Geometry check sheet. Reference: the model listing, model coordinates, mm. Face numbers are marked on the shaded views. A direction names the side the tool comes from. Coordinates: 2 decimals unless noted, no trailing zeros. Order: outer loops, then holes, each group sorted by start corner. A loop starts at its lowest first (then second) coordinate and runs counter-clockwise, first axis right, second up. Notation, with made-up numbers: (63, -14.5) - (72, -14.5) arc R28 ccw to (72, 22.5) - close; hole circle Ø10 at (26.25, 68.25). An arc over 180 degrees is marked (long way). Return JSON: item names as keys, results as strings. Group by question number.
Item 1: Section check C-C on z = 24.5. Enter the section's corners in (x, y), then the cut area to 3 significant figures.
Item 2: Section check A-A on y = -39.5. Enter the section's corners in (x, z).
Item 3: Tool access check on the marked faces 4, 5, 6, 7 and 8. Record the directions out of +Z, -Z, +X, -X, +Y, -Y that give a thin tool (end or side, any length) a straight path to the whole face; none if there is none.
Item 4: Draft check along Z on the marked faces 1, 2 and 3. Enter one of: pulls with the +Z half, pulls with the -Z half, needs draft (parallel to the pull), parting line crosses it, or undercut.
Item 5: Gauge pin test, flat ends, axial feed: pin 1 (4 mm diameter, centred on y = -45.5, z = 1, fed in from +X); pin 2 (6 mm diameter, centred on x = 35.5, z = 10, fed in from +Y); pin 3 (7.5 mm diameter, centred on y = -35.5, z = 40.5, fed in from +X); pin 4 (7.5 mm diameter, centred on x = 36, y = -36.5, fed in from +Z). Record the tip position at first contact, or that the pin passes through.
Item 6: Section check B-B on x = 27. Enter the section's corners in (y, z).
Item 7: Scan lines: probe 1 along X at (y, z) = (-31, 33); probe 2 along Z at (x, y) = (37, -11); probe 3 along Z at (x, y) = (7, -4). Record each from-to range of solid material in increasing order.
Item 8: Section check D-D on z = 45. Enter the section's corners in (x, y), then the cut area to 3 significant figures.
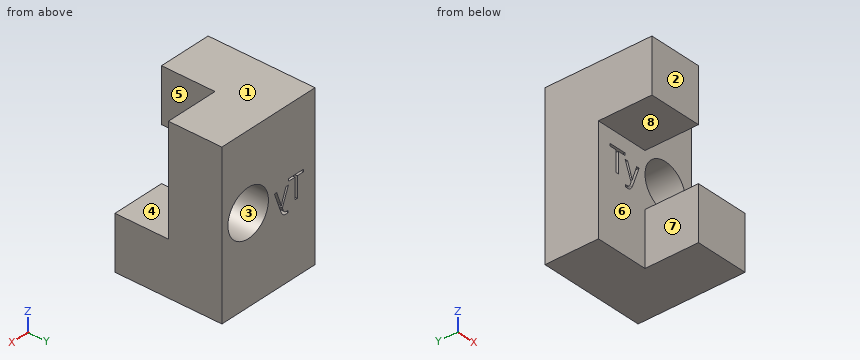
from build123d import *

# Parameters (mm, degrees)
F0_W     = 25.4
F0_H     = 25.4
F1_DEPTH = 50.8
F2_R     = 11.0649221301
F3_DEPTH = 25.4
F4_W     = 25.4
F4_H     = 25.4
F5_DEPTH = 50.8


with BuildPart() as f1:
    # F0 (on Front) → F1 (new body)
    with BuildSketch(Plane.XZ):
        with Locations((38.1, -12.7)):
            Rectangle(F0_W, F0_H)
    extrude(amount=F1_DEPTH)

    # F2 (on Front) → F3 (join)
    with BuildSketch(Plane.XZ):
        Polygon((0, 0), (0, -25.4), (25.4, -25.4), (25.4, 0), (50.8, 0), (50.8, 25.4), (50.8, 50.8), (25.4, 50.8), (25.4, 25.4), (0, 25.4), align=None)
        with BuildLine():
            Line((17.8367029688, 7.9644425954), (14.5494888325, 16.1563134241))
            Line((14.5494888325, 16.1563134241), (15.8743645734, 16.1563134241))
            Line((15.8743645734, 16.1563134241), (17.6583085692, 11.5109232591))
            add(Edge.make_bspline(
                [(17.6583085692, 11.5109232591), (18.2434421998, 9.9196452148), (18.3861577195, 9.2132033925)],
                knots=[0, 0, 0, 1, 1, 1], degree=2))
            Line((18.3861577195, 9.2132033925), (18.4456225193, 9.2132033925))
            add(Edge.make_bspline(
                [(18.4456225193, 9.2132033925), (18.5407661991, 9.5937781116), (18.8499831584, 10.5119146214)],
                knots=[0, 0, 0, 1, 1, 1], degree=2))
            add(Edge.make_bspline(
                [(18.8499831584, 10.5119146214), (19.1592001176, 11.4300511313), (20.8694077616, 16.1563134241)],
                knots=[0, 0, 0, 1, 1, 1], degree=2))
            Line((20.8694077616, 16.1563134241), (22.1919049105, 16.1563134241))
            Line((22.1919049105, 16.1563134241), (18.6906174947, 6.879804646))
            add(Edge.make_bspline(
                [(18.6906174947, 6.879804646), (18.169705848, 5.5049784733), (17.4751569856, 4.9281699146)],
                knots=[0, 0, 0, 1, 1, 1], degree=2))
            add(Edge.make_bspline(
                [(17.4751569856, 4.9281699146), (16.7806081233, 4.351361356), (15.7697065256, 4.351361356)],
                knots=[0, 0, 0, 1, 1, 1], degree=2))
            add(Edge.make_bspline(
                [(15.7697065256, 4.351361356), (15.203601631, 4.351361356), (14.6541468803, 4.4798053237)],
                knots=[0, 0, 0, 1, 1, 1], degree=2))
            Line((14.6541468803, 4.4798053237), (14.6541468803, 5.4669210013))
            add(Edge.make_bspline(
                [(14.6541468803, 5.4669210013), (15.0632647033, 5.3789130976), (15.5675262061, 5.3789130976)],
                knots=[0, 0, 0, 1, 1, 1], degree=2))
            add(Edge.make_bspline(
                [(15.5675262061, 5.3789130976), (16.8400729231, 5.3789130976), (17.3823918978, 6.8060682942)],
                knots=[0, 0, 0, 1, 1, 1], degree=2))
            Line((17.3823918978, 6.8060682942), (17.8367029688, 7.9644425954))
        make_face(mode=Mode.SUBTRACT)
        Polygon((10.950679145, 17.7547272443), (10.950679145, 8.0096358433), (9.687646796, 8.0096358433), (9.687646796, 17.7547272443), (6.2458241801, 17.7547272443), (6.2458241801, 18.8774226657), (14.3925017609, 18.8774226657), (14.3925017609, 17.7547272443), align=None, mode=Mode.SUBTRACT)
        with Locations((36.4649221301, 15.1761500165)):
            Circle(F2_R, mode=Mode.SUBTRACT)
    extrude(amount=F3_DEPTH)

    # F4 (on Front) → F5 (join)
    with BuildSketch(Plane.XZ):
        with Locations((12.7, 38.1)):
            Rectangle(F4_W, F4_H)
    extrude(amount=F5_DEPTH)


solid = f1.part
Computed:
{
 "1": {"outline": "(0, -25.4) - (30.51, -25.4) - (30.51, 0) - (0, 0) - close; (42.42, -25.4) - (50.8, -25.4) - (50.8, 0) - (42.42, 0) - close", "area": "988 mm²"},
 "2": {"outline": "(0, 25.4) - (25.4, 25.4) - (25.4, 50.8) - (0, 50.8) - close; (25.4, -25.4) - (50.8, -25.4) - (50.8, 0) - (25.4, 0) - close"},
 "3": {"face 4": "+Z, +X, -X, -Y", "face 5": "+Z, +X, -Y", "face 6": "-Y", "face 7": "-Z, -X, -Y", "face 8": "-Z, +X, -X, -Y"},
 "4": {"face 1": "pulls with the +Z half", "face 2": "needs draft", "face 3": "undercut"},
 "5": {"pin 1": "stops at x = 50.8", "pin 2": "passes through", "pin 3": "stops at x = 25.4", "pin 4": "stops at z = 0"},
 "6": {"outline": "(-50.8, -25.4) - (0, -25.4) - (0, 9.44) - (-25.4, 9.44) - (-25.4, 0) - (-50.8, 0) - close; (-25.4, 20.91) - (0, 20.91) - (0, 50.8) - (-25.4, 50.8) - close"},
 "7": {"probe 1": "x = 0 to 25.4", "probe 2": "z = -25.4 to 4.12, 26.23 to 50.8", "probe 3": "z = -25.4 to 17.75, 18.88 to 50.8"},
 "8": {"outline": "(0, -50.8) - (25.4, -50.8) - (25.4, -25.4) - (50.8, -25.4) - (50.8, 0) - (0, 0) - close", "area": "1,940 mm²"}
}
